Verification items for this drawing (mm, ordinates from the low corner). A direction names the side the tool comes from. Give positions to 0.01 mm unless a question says otherwise; leave off trailing zeros. Loops run counter-clockwise (first coordinate to the right, second up) from the corner with the lowest first, then second, coordinate; pieces in that order, holes last. Notation, with made-up numbers: (-1.5, -16) -> (47.5, -16) arc R33 cw to (47.5, 13) -> close; hole circle Ø10 at (29.5, 85). An arc over 180 degrees is marked (long way). Answer as CSV lines item,"result". Start each with the question number.
(1) Access from +Z, -Z, +X, -X, +Y, -Y to the whole of each face (thin tool, end or side, straight path). Record for the marked faces 1 and 2.
(2) Gauge pin test, flat end, axial feed: pin 1 Ø1.5 at (x, z) = (3, 4.5) entering from -Y. Record the tip position at first contact, or that the pin passes through.
(3) Material ranges on line 1 (Y direction, x = 10, z = 2.75); line 2 (Z direction, x = 19.25, y = 9.75); line 3 (Y direction, x = 14.25, z = 1.25), recorded low to high. Write a range as from..to.
(4) Section check C-C on z = 6. Enter the section's corners in (x, y).
(5) Section check A-A on y = 10. Enter the section's corners in (x, z), plus the area to 3 significant figures.
(6) Section check D-D on x = 1.5. Enter the section's corners in (y, z), plus the area to 3 significant figures.
(7) Release check for a two-part mould opening along Z. For the marked faces 3, 4 and 5 record: pulls with the +Z half, pulls with the -Z half, needs draft (parallel to the pull), parting line crosses it, or undercut.
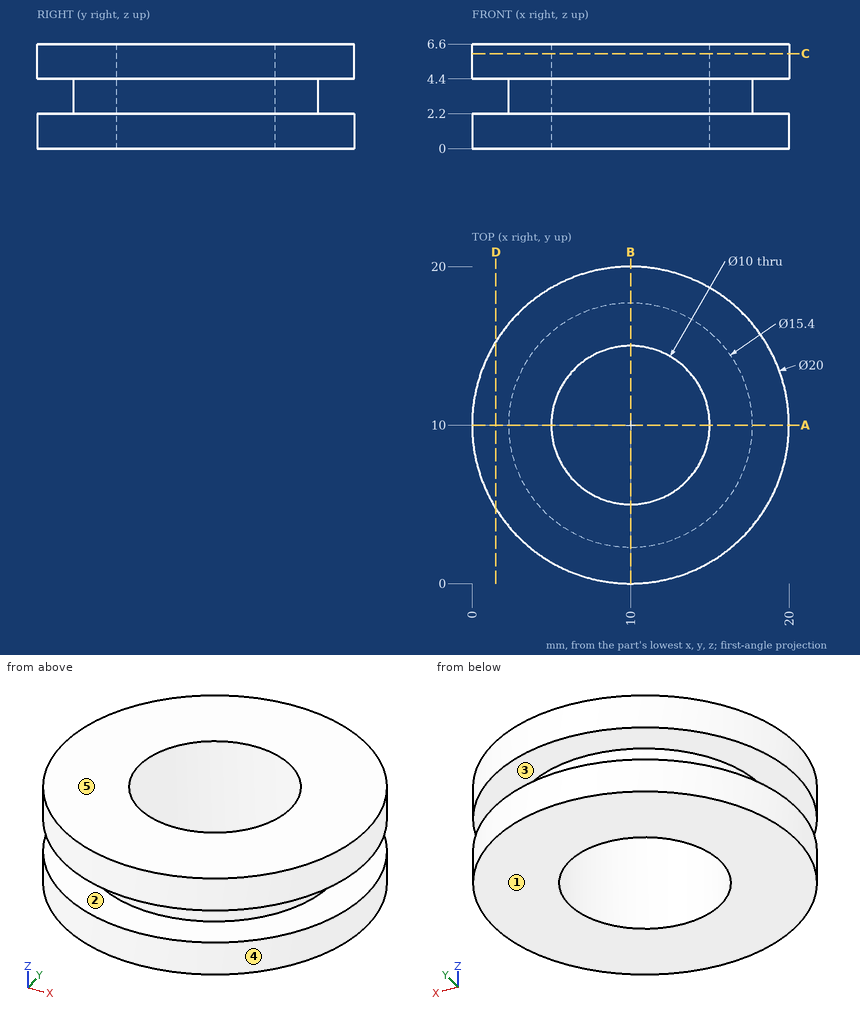
Working result:
1,face 1,"-Z, +X, -X, +Y, -Y"
1,face 2,"none"
2,pin 1,"stops at y = 2.19"
3,line 1,"y = 2.3..5, 15..17.7"
3,line 2,"z = 0..2.2, 4.4..6.6"
3,line 3,"y = 0.95..7.37, 12.63..19.05"
4,outline,"circle Ø20 at (10, 10); hole circle Ø10 at (10, 10)"
5,outline,"(0, 0) -> (5, 0) -> (5, 6.6) -> (0, 6.6) -> (0, 4.4) -> (2.3, 4.4) -> (2.3, 2.2) -> (0, 2.2) -> close; (15, 0) -> (20, 0) -> (20, 2.2) -> (17.7, 2.2) -> (17.7, 4.4) -> (20, 4.4) -> (20, 6.6) -> (15, 6.6) -> close"
5,area,"55.9 mm^2"
6,outline,"(4.73, 0) -> (15.27, 0) -> (15.27, 2.2) -> (4.73, 2.2) -> close; (4.73, 4.4) -> (15.27, 4.4) -> (15.27, 6.6) -> (4.73, 6.6) -> close"
6,area,"46.4 mm^2"
7,face 3,"undercut"
7,face 4,"needs draft"
7,face 5,"pulls with the +Z half"
